The listing builds one solid part. Answer for the finished solid, in the listing's coordinates (mm). A direction names the side the tool comes from. Round coordinates to 2 decimals unless told otherwise and drop trailing zeros. Order: outer loops, then holes, each group sorted by start corner. A loop starts at its lowest first (then second) coordinate and runs counter-clockwise, first axis right, second up. Notation, with made-up numbers: M 45,-18 L 53,-18 A31 cw 53,20 Z; hole C -17.75,6.25 d3. An arc over 180 degrees is marked long. Write item = value, one per line. Start each with the question number.
(1) Each of these flat-tipped pins is pushed along its axis until it touches: pin 1 (6 mm diameter, centred on x = 6, z = -12.5, fed in from +Y); pin 2 (9.5 mm diameter, centred on x = 23, z = -12.5, fed in from +Y); pin 3 (2.5 mm diameter, centred on x = 54, z = -12.5, fed in from +Y). Where does it stop, or does it pass through?
(2) A cutting plane is placed at A-A, the plane y = 9.5. Determine the outline of the cut face in (x, z), and give its area (3 significant figures).
(3) Straight lines are drawn through the part: probe 1 along X at (y, z) = (8.5, -12.5); probe 2 along X at (y, z) = (3.5, -12.5); probe 3 along Y at (x, z) = (36, -10.25). For each, find the intervals that lie inside material, in ascending order. Write a range as from..to.
(4) Which of the six approach directions +Z, -Z, +X, -X, +Y, -Y give full straight-line access (tool end or side, diameter ignored) to faces 1 (the face through (48.36, 11.45, -0.9)), 2 (the face through (30, 5, -13)), 3 (the face through (30.203, 4.31, -23.914))?
(5) A cutting plane is placed at D-D, the plane x = 39. Determine the outline of the cut face in (y, z), and give its area (3 significant figures).
(6) A cutting plane is placed at C-C, the plane x = 6. Determine the outline of the cut face in (y, z), and give its area (3 significant figures).
(7) For a pull along X with two mould halves and no side action, classify faces 4 (the face through (11.6, 11.45, -0.86)), 5 (the face through (0.86, 9.08, -24.1)), 6 (the face through (60, 9, -12)) as released by +X, released by -X, zero draft, split by the parting line, or undercut.
(8) A cutting plane is placed at B-B, the plane z = -12.5. Determine the outline of the cut face in (x, y), and give its area (3 significant figures).
from build123d import *

# Parameters (mm, degrees)
SKETCH1_W           = 60
SKETCH1_H           = 25
BOSS_EXTRUDE1_DEPTH = 5
SKETCH2_W           = 12.5
SKETCH2_H           = 25
BOSS_EXTRUDE2_DEPTH = 10
SKETCH3_R           = 2.25
CUT_EXTRUDE1_DEPTH  = 15
FILLET1_R           = 3


with BuildPart() as part:
    # Sketch1 → Boss-Extrude1 (new body)
    with BuildSketch(Plane(origin=(0, 0, 0), x_dir=(1, 0, 0), z_dir=(0, 1, 0))):
        with Locations((30, 12.5)):
            Rectangle(SKETCH1_W, SKETCH1_H)
    extrude(amount=BOSS_EXTRUDE1_DEPTH)

    # Sketch2 → Boss-Extrude2 (add)
    with BuildSketch(Plane(origin=(0, 5, 0), x_dir=(1, 0, 0), z_dir=(0, 1, 0))):
        with Locations((6.25, 12.5)):
            Rectangle(SKETCH2_W, SKETCH2_H)
        with Locations((53.75, 12.5)):
            Rectangle(SKETCH2_W, SKETCH2_H)
    extrude(amount=BOSS_EXTRUDE2_DEPTH)

    # Sketch3 → Cut-Extrude1 (cut)
    with BuildSketch(Plane.XZ):
        with Locations(Location((6, -12.5, 0), (0, 0, 270))):
            Circle(SKETCH3_R)
        with Locations(Location((54, -12.5, 0), (0, 0, 90))):
            Circle(SKETCH3_R)
    extrude(amount=-CUT_EXTRUDE1_DEPTH, mode=Mode.SUBTRACT)

    # Fillet1
    # the kernel refuses this fillet: 3 mm, written as the material it adds along each edge
    with BuildSketch(Plane(origin=(12.5, 5, -25), x_dir=(0, 1, 0), z_dir=(0, 0, 1)), Plane(origin=(47.5, 5, -25), x_dir=(-1, 0, 0), z_dir=(0, 0, 1))) as fillet1_piece_1:
        with BuildLine():
            CenterArc((FILLET1_R, -FILLET1_R), FILLET1_R, 90, 90)
            Line((0, -FILLET1_R), (0, 0))
            Line((0, 0), (FILLET1_R, 0))
        make_face()
    extrude(amount=25)
    # the kernel refuses this fillet: 3 mm, written as the material it takes off along each edge
    with BuildSketch(Plane(origin=(57, 3, -22), x_dir=(0, 0, -1), z_dir=(0, -1, 0))) as fillet1_2_piece_1_section:
        Polygon((0, 0), (FILLET1_R * 1.02, 0), (FILLET1_R * 1.02, FILLET1_R * 1.02), (0, FILLET1_R * 1.02), align=None)
    fillet1_2_piece_1 = extrude(amount=FILLET1_R * 1.02, mode=Mode.PRIVATE)
    fillet1_2_piece_1 = fillet1_2_piece_1 - Plane(origin=(57, 3, -22), x_dir=(-0.7071067811865475, 0, 0.7071067811865475), z_dir=(0, -1, 0)) * Sphere(FILLET1_R, mode=Mode.PRIVATE)
    add(fillet1_2_piece_1, mode=Mode.SUBTRACT)
    with BuildSketch(Plane(origin=(3, 3, -22), x_dir=(0, 0, -1), z_dir=(0, -1, 0))) as fillet1_2_piece_2_section:
        Polygon((0, 0), (FILLET1_R * 1.02, 0), (FILLET1_R * 1.02, -FILLET1_R * 1.02), (0, -FILLET1_R * 1.02), align=None)
    fillet1_2_piece_2 = extrude(amount=FILLET1_R * 1.02, mode=Mode.PRIVATE)
    fillet1_2_piece_2 = fillet1_2_piece_2 - Plane(origin=(3, 3, -22), x_dir=(0.7071067811865475, 0, 0.7071067811865475), z_dir=(0, -1, 0)) * Sphere(FILLET1_R, mode=Mode.PRIVATE)
    add(fillet1_2_piece_2, mode=Mode.SUBTRACT)
    with BuildSketch(Plane(origin=(57, 3, -3), x_dir=(0, 0, 1), z_dir=(0, -1, 0))) as fillet1_2_piece_3_section:
        Polygon((0, 0), (FILLET1_R * 1.02, 0), (FILLET1_R * 1.02, -FILLET1_R * 1.02), (0, -FILLET1_R * 1.02), align=None)
    fillet1_2_piece_3 = extrude(amount=FILLET1_R * 1.02, mode=Mode.PRIVATE)
    fillet1_2_piece_3 = fillet1_2_piece_3 - Plane(origin=(57, 3, -3), x_dir=(-0.7071067811865475, 0, -0.7071067811865475), z_dir=(0, -1, 0)) * Sphere(FILLET1_R, mode=Mode.PRIVATE)
    add(fillet1_2_piece_3, mode=Mode.SUBTRACT)
    with BuildSketch(Plane(origin=(3, 3, -3), x_dir=(0, -1, 0), z_dir=(0, 0, 1))) as fillet1_2_piece_4_section:
        Polygon((0, 0), (FILLET1_R * 1.02, 0), (FILLET1_R * 1.02, -FILLET1_R * 1.02), (0, -FILLET1_R * 1.02), align=None)
    fillet1_2_piece_4 = extrude(amount=FILLET1_R * 1.02, mode=Mode.PRIVATE)
    fillet1_2_piece_4 = fillet1_2_piece_4 - Plane(origin=(3, 3, -3), x_dir=(0.7071067811865475, 0.7071067811865475, 0), z_dir=(0, 0, 1)) * Sphere(FILLET1_R, mode=Mode.PRIVATE)
    add(fillet1_2_piece_4, mode=Mode.SUBTRACT)
    with BuildSketch(Plane(origin=(57, 0, -25), x_dir=(0, 0, 1), z_dir=(-1, 0, 0))) as fillet1_2_piece_5:
        with BuildLine():
            CenterArc((FILLET1_R, FILLET1_R), FILLET1_R, 180, 90)
            Line((0, FILLET1_R), (0, 0))
            Line((0, 0), (FILLET1_R, 0))
        make_face()
    extrude(amount=54, mode=Mode.SUBTRACT)
    with BuildSketch(Plane(origin=(60, 0, -3), x_dir=(0, 1, 0), z_dir=(0, 0, -1)), Plane(origin=(0, 0, -22), x_dir=(0, 1, 0), z_dir=(0, 0, 1))) as fillet1_2_piece_6:
        with BuildLine():
            CenterArc((FILLET1_R, -FILLET1_R), FILLET1_R, 90, 90)
            Line((0, -FILLET1_R), (0, 0))
            Line((0, 0), (FILLET1_R, 0))
        make_face()
    extrude(amount=19, mode=Mode.SUBTRACT)
    with BuildSketch(Plane(origin=(3, 0, 0), x_dir=(0, 1, 0), z_dir=(1, 0, 0))) as fillet1_2_piece_7:
        with BuildLine():
            CenterArc((FILLET1_R, -FILLET1_R), FILLET1_R, 90, 90)
            Line((0, -FILLET1_R), (0, 0))
            Line((0, 0), (FILLET1_R, 0))
        make_face()
    extrude(amount=54, mode=Mode.SUBTRACT)
    with BuildSketch(Plane(origin=(0, 22.5, -25), x_dir=(0, 0, 1), z_dir=(0, -1, 0)), Plane(origin=(60, 3, -25), x_dir=(0, 0, 1), z_dir=(0, 1, 0)), Plane(origin=(60, 3, 0), x_dir=(-1, 0, 0), z_dir=(0, 1, 0)), Plane(origin=(0, 22.5, 0), x_dir=(1, 0, 0), z_dir=(0, -1, 0))) as fillet1_2_piece_8:
        with BuildLine():
            CenterArc((FILLET1_R, -FILLET1_R), FILLET1_R, 90, 90)
            Line((0, -FILLET1_R), (0, 0))
            Line((0, 0), (FILLET1_R, 0))
        make_face()
    extrude(amount=19.5, mode=Mode.SUBTRACT)
    # the kernel refuses this fillet: 3 mm, written as the material it takes off along each edge
    with BuildSketch(Plane(origin=(15.5, 5, 0), x_dir=(0, -1, 0), z_dir=(1, 0, 0))) as fillet1_3_piece_1:
        with BuildLine():
            CenterArc((FILLET1_R, FILLET1_R), FILLET1_R, 180, 90)
            Line((0, FILLET1_R), (0, 0))
            Line((0, 0), (FILLET1_R, 0))
        make_face()
    extrude(amount=29, mode=Mode.SUBTRACT)
    with BuildSketch(Plane(origin=(12.5, 8, 0), x_dir=(-1, 0, 0), z_dir=(0, 1, 0)), Plane(origin=(12.5, 8, -25), x_dir=(0, 0, 1), z_dir=(0, 1, 0))) as fillet1_3_piece_2:
        with BuildLine():
            CenterArc((FILLET1_R, -FILLET1_R), FILLET1_R, 90, 90)
            Line((0, -FILLET1_R), (0, 0))
            Line((0, 0), (FILLET1_R, 0))
        make_face()
    extrude(amount=14.5, mode=Mode.SUBTRACT)
    with BuildSketch(Plane(origin=(44.5, 5, -25), x_dir=(0, 0, 1), z_dir=(-1, 0, 0))) as fillet1_3_piece_3:
        with BuildLine():
            CenterArc((FILLET1_R, -FILLET1_R), FILLET1_R, 90, 90)
            Line((0, -FILLET1_R), (0, 0))
            Line((0, 0), (FILLET1_R, 0))
        make_face()
    extrude(amount=29, mode=Mode.SUBTRACT)
    with BuildSketch(Plane(origin=(47.5, 8, -25), x_dir=(0, 0, 1), z_dir=(0, 1, 0)), Plane(origin=(47.5, 8, 0), x_dir=(1, 0, 0), z_dir=(0, 1, 0))) as fillet1_3_piece_4:
        with BuildLine():
            CenterArc((FILLET1_R, FILLET1_R), FILLET1_R, 180, 90)
            Line((0, FILLET1_R), (0, 0))
            Line((0, 0), (FILLET1_R, 0))
        make_face()
    extrude(amount=14.5, mode=Mode.SUBTRACT)
    with BuildSketch(Plane(origin=(44.5, 8, 0), x_dir=(0, -1, 0), z_dir=(-1, 0, 0))) as fillet1_3_piece_5:
        with BuildLine():
            CenterArc((3 + FILLET1_R, -FILLET1_R), FILLET1_R, 90, 90)
            Line((3, -FILLET1_R), (3, 0))
            Line((3, 0), (3 + FILLET1_R, 0))
        make_face()
    revolve(axis=Axis((44.5, 8, 0), (0, 0, 1)), revolution_arc=90, mode=Mode.SUBTRACT)
    with BuildSketch(Plane(origin=(44.5, 8, -25), x_dir=(0, -1, 0), z_dir=(-1, 0, 0))) as fillet1_3_piece_6:
        with BuildLine():
            CenterArc((3 + FILLET1_R, FILLET1_R), FILLET1_R, 180, 90)
            Line((3 + FILLET1_R, 0), (3, 0))
            Line((3, 0), (3, FILLET1_R))
        make_face()
    revolve(axis=Axis((44.5, 8, -25), (0, 0, 1)), revolution_arc=90, mode=Mode.SUBTRACT)
    with BuildSketch(Plane(origin=(15.5, 8, -25), x_dir=(-1, 0, 0), z_dir=(0, 1, 0))) as fillet1_3_piece_7:
        with BuildLine():
            CenterArc((3 + FILLET1_R, FILLET1_R), FILLET1_R, 180, 90)
            Line((3 + FILLET1_R, 0), (3, 0))
            Line((3, 0), (3, FILLET1_R))
        make_face()
    revolve(axis=Axis((15.5, 8, -25), (0, 0, 1)), revolution_arc=90, mode=Mode.SUBTRACT)
    with BuildSketch(Plane(origin=(15.5, 8, 0), x_dir=(-1, 0, 0), z_dir=(0, 1, 0))) as fillet1_3_piece_8:
        with BuildLine():
            CenterArc((3 + FILLET1_R, -FILLET1_R), FILLET1_R, 90, 90)
            Line((3, -FILLET1_R), (3, 0))
            Line((3, 0), (3 + FILLET1_R, 0))
        make_face()
    revolve(axis=Axis((15.5, 8, 0), (0, 0, 1)), revolution_arc=90, mode=Mode.SUBTRACT)


solid = part.part
Reported:
q1.pin_1 = 15
q1.pin_2 = 5
q1.pin_3 = through
q2.outline = M 0,-22 A3 ccw 3,-25 L 9.5,-25 A3 ccw 12.5,-22 L 12.5,-3 A3 ccw 9.5,0 L 3,0 A3 ccw 0,-3 Z; M 47.5,-22 A3 ccw 50.5,-25 L 57,-25 A3 ccw 60,-22 L 60,-3 A3 ccw 57,0 L 50.5,0 A3 ccw 47.5,-3 Z; hole C 6,-12.5 d4.5; hole C 54,-12.5 d4.5
q2.area = 578 mm²
q3.probe_1 = 0..3.75, 8.25..12.5, 47.5..51.75, 56.25..60
q3.probe_2 = 0..3.75, 8.25..51.75, 56.25..60
q3.probe_3 = 0..5
q4.face_1 = +Z, +Y
q4.face_2 = +Z, -Z, +Y
q4.face_3 = -Z, +Y
q5.outline = M 0,-22 A3 ccw 2.5,-24.96 A3 ccw 5,-22 L 5,-3 A3 ccw 2.5,-0.04 A3 ccw 0,-3 Z
q5.area = 117 mm²
q6.outline = M 0,-22 A3 ccw 3,-25 L 15,-25 L 15,-14.75 L 0,-14.75 Z; M 0,-10.25 L 15,-10.25 L 15,0 L 3,0 A3 ccw 0,-3 Z
q6.area = 304 mm²
q7.face_4 = undercut
q7.face_5 = released by -X
q7.face_6 = released by +X
q8.outline = M 0,3 A3 ccw 3,0 L 3.75,0 L 3.75,15 L 0,15 Z; M 8.25,0 L 51.75,0 L 51.75,15 L 47.5,15 L 47.5,8 A3 cw 44.5,5 L 15.5,5 A3 cw 12.5,8 L 12.5,15 L 8.25,15 Z; M 56.25,0 L 57,0 A3 ccw 60,3 L 60,15 L 56.25,15 Z
q8.area = 415 mm²
